The model under review builds one solid part; all positions refer to its coordinate system, in mm. Coordinates: 2 decimals unless noted, no trailing zeros. Order: outer loops, then holes, each group sorted by start corner. A loop starts at its lowest first (then second) coordinate and runs counter-clockwise, first axis right, second up. Notation, with made-up numbers: (-28.75, -37.5) -> (-10.75, -37.5) arc R25 ccw to (-10.75, -1.5) -> close; hole circle Ø5 at (1.5, 3). An arc over 180 degrees is marked (long way). Put each result on its own line as item: value.
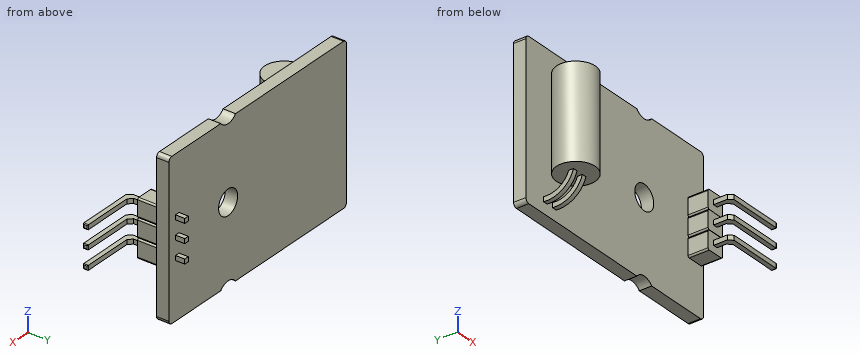
from build123d import *

# Parameters (mm, degrees)
BOX214_W                  = 0.6
BOX214_H                  = 0.6
BOX214_DEPTH              = 7.7
BOX213_W                  = 0.6
BOX213_H                  = 0.6
BOX213_DEPTH              = 7.7
CHAMFER002_SIZE           = 0.5
CHAMFER003_SIZE           = 0.5
FILLET164_R               = 0.1
BOX212_W                  = 2.4
BOX212_H                  = 2.4
BOX212_DEPTH              = 2.6
FILLET163_R               = 0.2
BOX217_W                  = 0.6
BOX217_H                  = 0.6
BOX217_DEPTH              = 7.7
BOX216_W                  = 0.6
BOX216_H                  = 0.6
BOX216_DEPTH              = 7.7
CHAMFER004_SIZE           = 0.5
CHAMFER005_SIZE           = 0.5
FILLET166_R               = 0.1
BOX215_W                  = 2.4
BOX215_H                  = 2.4
BOX215_DEPTH              = 2.6
FILLET165_R               = 0.2
BOX220_W                  = 0.6
BOX220_H                  = 0.6
BOX220_DEPTH              = 7.7
BOX219_W                  = 0.6
BOX219_H                  = 0.6
BOX219_DEPTH              = 7.7
CHAMFER006_SIZE           = 0.5
CHAMFER007_SIZE           = 0.5
FILLET168_R               = 0.1
BOX218_W                  = 2.4
BOX218_H                  = 2.4
BOX218_DEPTH              = 2.6
FILLET167_R               = 0.2
BOX221_W                  = 10
BOX221_H                  = 10
BOX221_DEPTH              = 10
BOX222_W                  = 10
BOX222_H                  = 10
BOX222_DEPTH              = 10
TUBE003_R                 = 3.6
TUBE003_R_2               = 3
TUBE003_DEPTH             = 0.6
TUBE004_R                 = 3.6
TUBE004_R_2               = 3
TUBE004_DEPTH             = 0.6
CYLINDER193_R             = 2
CYLINDER193_DEPTH         = 1
CYLINDER194_R             = 2
CYLINDER194_DEPTH         = 1
CYLINDER192_R             = 2.5
CYLINDER192_DEPTH         = 12
FUSION007_PLACEMENT_ANGLE = 90
CYLINDER191_R             = 1.6
CYLINDER191_DEPTH         = 10
CYLINDER001_R             = 1.6
CYLINDER001_DEPTH         = 10
CYLINDER190_R             = 1.6
CYLINDER190_DEPTH         = 10
BOX211_W                  = 30
BOX211_H                  = 20
BOX211_DEPTH              = 1.6
FILLET161_R               = 0.5
FILLET162_R               = 0.5
FUSION010_PLACEMENT_ANGLE = 90


with BuildPart() as cubo201:
    # Box214 → Box214 (new body)
    with BuildSketch(Plane(origin=(0, 0, 7.7), x_dir=(0, 0, -1), z_dir=(1, 0, 0))):
        with Locations((0.3, 0.3)):
            Rectangle(BOX214_W, BOX214_H)
    extrude(amount=BOX214_DEPTH)


with BuildPart() as cuerpometal:
    # Box213 → Box213 (new body)
    with BuildSketch(Plane.XY):
        with Locations((0.3, 0.3)):
            Rectangle(BOX213_W, BOX213_H)
    extrude(amount=BOX213_DEPTH)

    # Fusion139: union Cubo201
    add(cubo201.part)

    # Chamfer002
    chamfer002_edges = [cuerpometal.edges().sort_by_distance(p)[0] for p in [
        (0, 0.3, 7.7),
    ]]
    chamfer(chamfer002_edges, length=CHAMFER002_SIZE)

    # Chamfer003
    chamfer003_edges = [cuerpometal.edges().sort_by_distance(p)[0] for p in [
        (0.6, 0.3, 7.1),
    ]]
    chamfer(chamfer003_edges, length=CHAMFER003_SIZE)

    # Fillet164
    fillet164_edges = [cuerpometal.edges().sort_by_distance(p)[0] for p in [
        (7.7, 0, 7.4),
        (7.7, 0.3, 7.1),
        (7.7, 0.3, 7.7),
        (7.7, 0.6, 7.4),
    ]]
    fillet(fillet164_edges, radius=FILLET164_R)


with BuildPart() as cuerpometal_1:
    # Fillet164 placement: moved
    add(cuerpometal.part.moved(Location((0.9, 0.9, -1.2))))


with BuildPart() as obj1:
    # Box212 → Box212 (new body)
    with BuildSketch(Plane.XY.offset(1.6)):
        with Locations((1.2, 1.2)):
            Rectangle(BOX212_W, BOX212_H)
    extrude(amount=BOX212_DEPTH)

    # Fillet163
    fillet163_edges = [obj1.edges().sort_by_distance(p)[0] for p in [
        (0, 0, 2.9),
        (0, 2.4, 2.9),
        (2.4, 0, 2.9),
        (2.4, 2.4, 2.9),
    ]]
    fillet(fillet163_edges, radius=FILLET163_R)

    # Fusion001: union CuerpoMetal
    add(cuerpometal_1.part)


with BuildPart() as obj1_1:
    # Fusion001 placement: moved
    add(obj1.part.moved(Location((12.4, -1.2, 0))))


with BuildPart() as cubo204:
    # Box217 → Box217 (new body)
    with BuildSketch(Plane(origin=(0, 0, 7.7), x_dir=(0, 0, -1), z_dir=(1, 0, 0))):
        with Locations((0.3, 0.3)):
            Rectangle(BOX217_W, BOX217_H)
    extrude(amount=BOX217_DEPTH)


with BuildPart() as cuerpometal001:
    # Box216 → Box216 (new body)
    with BuildSketch(Plane.XY):
        with Locations((0.3, 0.3)):
            Rectangle(BOX216_W, BOX216_H)
    extrude(amount=BOX216_DEPTH)

    # Fusion140: union Cubo204
    add(cubo204.part)

    # Chamfer004
    chamfer004_edges = [cuerpometal001.edges().sort_by_distance(p)[0] for p in [
        (0, 0.3, 7.7),
    ]]
    chamfer(chamfer004_edges, length=CHAMFER004_SIZE)

    # Chamfer005
    chamfer005_edges = [cuerpometal001.edges().sort_by_distance(p)[0] for p in [
        (0.6, 0.3, 7.1),
    ]]
    chamfer(chamfer005_edges, length=CHAMFER005_SIZE)

    # Fillet166
    fillet166_edges = [cuerpometal001.edges().sort_by_distance(p)[0] for p in [
        (7.7, 0, 7.4),
        (7.7, 0.3, 7.1),
        (7.7, 0.3, 7.7),
        (7.7, 0.6, 7.4),
    ]]
    fillet(fillet166_edges, radius=FILLET166_R)


with BuildPart() as cuerpometal001_1:
    # Fillet166 placement: moved
    add(cuerpometal001.part.moved(Location((0.9, 0.9, -1.2))))


with BuildPart() as obj2:
    # Box215 → Box215 (new body)
    with BuildSketch(Plane.XY.offset(1.6)):
        with Locations((1.2, 1.2)):
            Rectangle(BOX215_W, BOX215_H)
    extrude(amount=BOX215_DEPTH)

    # Fillet165
    fillet165_edges = [obj2.edges().sort_by_distance(p)[0] for p in [
        (0, 0, 2.9),
        (0, 2.4, 2.9),
        (2.4, 0, 2.9),
        (2.4, 2.4, 2.9),
    ]]
    fillet(fillet165_edges, radius=FILLET165_R)

    # Fusion003: union CuerpoMetal001
    add(cuerpometal001_1.part)


with BuildPart() as obj2_1:
    # Fusion003 placement: moved
    add(obj2.part.moved(Location((12.4, 1.22, 0))))


with BuildPart() as cubo207:
    # Box220 → Box220 (new body)
    with BuildSketch(Plane(origin=(0, 0, 7.7), x_dir=(0, 0, -1), z_dir=(1, 0, 0))):
        with Locations((0.3, 0.3)):
            Rectangle(BOX220_W, BOX220_H)
    extrude(amount=BOX220_DEPTH)


with BuildPart() as cuerpometal002:
    # Box219 → Box219 (new body)
    with BuildSketch(Plane.XY):
        with Locations((0.3, 0.3)):
            Rectangle(BOX219_W, BOX219_H)
    extrude(amount=BOX219_DEPTH)

    # Fusion004: union Cubo207
    add(cubo207.part)

    # Chamfer006
    chamfer006_edges = [cuerpometal002.edges().sort_by_distance(p)[0] for p in [
        (0, 0.3, 7.7),
    ]]
    chamfer(chamfer006_edges, length=CHAMFER006_SIZE)

    # Chamfer007
    chamfer007_edges = [cuerpometal002.edges().sort_by_distance(p)[0] for p in [
        (0.6, 0.3, 7.1),
    ]]
    chamfer(chamfer007_edges, length=CHAMFER007_SIZE)

    # Fillet168
    fillet168_edges = [cuerpometal002.edges().sort_by_distance(p)[0] for p in [
        (7.7, 0, 7.4),
        (7.7, 0.3, 7.1),
        (7.7, 0.3, 7.7),
        (7.7, 0.6, 7.4),
    ]]
    fillet(fillet168_edges, radius=FILLET168_R)


with BuildPart() as cuerpometal002_1:
    # Fillet168 placement: moved
    add(cuerpometal002.part.moved(Location((0.9, 0.9, -1.2))))


with BuildPart() as obj3:
    # Box218 → Box218 (new body)
    with BuildSketch(Plane.XY.offset(1.6)):
        with Locations((1.2, 1.2)):
            Rectangle(BOX218_W, BOX218_H)
    extrude(amount=BOX218_DEPTH)

    # Fillet167
    fillet167_edges = [obj3.edges().sort_by_distance(p)[0] for p in [
        (0, 0, 2.9),
        (0, 2.4, 2.9),
        (2.4, 0, 2.9),
        (2.4, 2.4, 2.9),
    ]]
    fillet(fillet167_edges, radius=FILLET167_R)

    # Fusion005: union CuerpoMetal002
    add(cuerpometal002_1.part)


with BuildPart() as obj3_1:
    # Fusion005 placement: moved
    add(obj3.part.moved(Location((12.4, -3.64, 0))))


with BuildPart() as cubo208:
    # Box221 → Box221 (new body)
    with BuildSketch(Plane(origin=(-14, -6, 0), x_dir=(1, 0, 0), z_dir=(0, 0, 1))):
        with Locations((5, 5)):
            Rectangle(BOX221_W, BOX221_H)
    extrude(amount=BOX221_DEPTH)


with BuildPart() as cubo011:
    # Box222 → Box222 (new body)
    with BuildSketch(Plane(origin=(-14, -11, -10), x_dir=(1, 0, 0), z_dir=(0, 0, 1))):
        with Locations((5, 5)):
            Rectangle(BOX222_W, BOX222_H)
    extrude(amount=BOX222_DEPTH)


with BuildPart() as tube003:
    # Tube003 → Tube003 (new body)
    with BuildSketch(Plane(origin=(-12, -5, 2), x_dir=(0, 0, -1), z_dir=(1, 0, 0))):
        Circle(TUBE003_R)
        Circle(TUBE003_R_2, mode=Mode.SUBTRACT)
    extrude(amount=TUBE003_DEPTH)


with BuildPart() as sensor:
    # Tube004 → Tube004 (new body)
    with BuildSketch(Plane(origin=(-10.5, -5, 2), x_dir=(0, 0, -1), z_dir=(1, 0, 0))):
        Circle(TUBE004_R)
        Circle(TUBE004_R_2, mode=Mode.SUBTRACT)
    extrude(amount=TUBE004_DEPTH)

    # Fusion008: union Tube003
    add(tube003.part)

    # Cut262: cut Cubo011
    add(cubo011.part, mode=Mode.SUBTRACT)

    # Cut263: cut Cubo208
    add(cubo208.part, mode=Mode.SUBTRACT)


with BuildPart() as cilindro193:
    # Cylinder193 → Cylinder193 (new body)
    with BuildSketch(Plane.XY):
        Circle(CYLINDER193_R)
    extrude(amount=CYLINDER193_DEPTH)


with BuildPart() as cilindro194:
    # Cylinder194 → Cylinder194 (new body)
    with BuildSketch(Plane.XY.offset(11)):
        Circle(CYLINDER194_R)
    extrude(amount=CYLINDER194_DEPTH)


with BuildPart() as fusion009:
    # Cylinder192 → Cylinder192 (new body)
    with BuildSketch(Plane.XY):
        Circle(CYLINDER192_R)
    extrude(amount=CYLINDER192_DEPTH)

    # Fusion006: union Cilindro194
    add(cilindro194.part)

    # Fusion007: union Cilindro193
    add(cilindro193.part)


with BuildPart() as fusion009_1:
    # Fusion007 placement: moved
    add(fusion009.part.moved(Location((-11, 6, 5))).rotate(Axis((-11, 6, 5), (1, 0, 0)), FUSION007_PLACEMENT_ANGLE))

    # Fusion009: union Sensor
    add(sensor.part)


with BuildPart() as cilindro191:
    # Cylinder191 → Cylinder191 (new body)
    with BuildSketch(Plane(origin=(5, 11, 0), x_dir=(1, 0, 0), z_dir=(0, 0, 1))):
        Circle(CYLINDER191_R)
    extrude(amount=CYLINDER191_DEPTH)


with BuildPart() as cilindro001:
    # Cylinder001 → Cylinder001 (new body)
    with BuildSketch(Plane(origin=(5, -11, 0), x_dir=(1, 0, 0), z_dir=(0, 0, 1))):
        Circle(CYLINDER001_R)
    extrude(amount=CYLINDER001_DEPTH)


with BuildPart() as cilindro190:
    # Cylinder190 → Cylinder190 (new body)
    with BuildSketch(Plane(origin=(5, 0, 0), x_dir=(1, 0, 0), z_dir=(0, 0, 1))):
        Circle(CYLINDER190_R)
    extrude(amount=CYLINDER190_DEPTH)


with BuildPart() as obj4:
    # Box211 → Box211 (new body)
    with BuildSketch(Plane.XY):
        with Locations((15, 10)):
            Rectangle(BOX211_W, BOX211_H)
    extrude(amount=BOX211_DEPTH)

    # Fillet161
    fillet161_edges = [obj4.edges().sort_by_distance(p)[0] for p in [
        (0, 0, 0.8),
        (0, 20, 0.8),
        (30, 20, 0.8),
    ]]
    fillet(fillet161_edges, radius=FILLET161_R)

    # Fillet162
    fillet162_edges = [obj4.edges().sort_by_distance(p)[0] for p in [
        (30, 0, 0.8),
    ]]
    fillet(fillet162_edges, radius=FILLET162_R)


with BuildPart() as obj4_1:
    # Fillet162 placement: moved
    add(obj4.part.moved(Location((-15, -10, 0))))

    # Cut259: cut Cilindro190
    add(cilindro190.part, mode=Mode.SUBTRACT)

    # Cut260: cut Cilindro001
    add(cilindro001.part, mode=Mode.SUBTRACT)

    # Cut261: cut Cilindro191
    add(cilindro191.part, mode=Mode.SUBTRACT)

    # Fusion010: union obj1, obj2, obj3, Fusion009
    add(obj1_1.part)
    add(obj2_1.part)
    add(obj3_1.part)
    add(fusion009_1.part)


with BuildPart() as obj4_2:
    # Fusion010 placement: moved
    add(obj4_1.part.moved(Location((0, 1, -0.6))).rotate(Axis((0, 1, -0.6), (1, 0, 0)), FUSION010_PLACEMENT_ANGLE))


solid = obj4_2.part
Item 1: Consider section B-B on z = 4.5. Write out the cut boundary in (x, y), and give its area (3 significant figures).
Answers below:
outline: (-15, -0.6) -> (15, -0.6) -> (15, 1) -> (-15, 1) -> close; circle Ø5 at (-11, -4)
area: 67.6 mm^2
Item 2: Consider section A-A on x = -11. Write out the cut boundary in (y, z), and give its area (3 significant figures).
Answers below:
outline: (-6.5, -6.6) -> (-1.5, -6.6) -> (-1.5, 5.4) -> (-6.5, 5.4) -> close; (-0.6, -10.6) -> (1, -10.6) -> (1, 9.4) -> (-0.6, 9.4) -> close
area: 92.0 mm^2
Item 3: For pin 1 Ø0.6 at (x, y) = (13.5, -2.5) entering from -Z; pin 2 Ø1.6 at (x, y) = (14, -1.5) entering from +Z; pin 3 Ø0.5 at (y, z) = (-4, 2) entering from +X; pin 4 Ø1.5 at (x, y) = (4, -2.5) entering from -Z, all flat-tipped, find the tip position at first contact; note any pin that passes through.
Answers below:
pin 1: z = -4.24
pin 2: z = 3.02
pin 3: x = 13.9
pin 4: through
Item 4: For line 1 (X direction, y = 0.3, z = -0.6); line 2 (Y direction, x = -1, z = 1); line 3 (X direction, y = 0, z = -3.5), list the stretches that pass through material, from the lowest coordinate up. Write a range as from..to.
Answers below:
line 1: -15..3.4, 6.6..15
line 2: -0.6..1
line 3: -15..15
Item 5: Consider section D-D on z = 7. Write out the cut boundary in (x, y).
Answers below:
outline: (-15, -0.6) -> (15, -0.6) -> (15, 1) -> (-15, 1) -> close
Item 6: Consider section C-C on x = 5. Write out the cut boundary in (y, z).
Answers below:
outline: (-0.6, -10) -> (1, -10) -> (1, -2.2) -> (-0.6, -2.2) -> close; (-0.6, 1) -> (1, 1) -> (1, 8.8) -> (-0.6, 8.8) -> close
